Autodesk Inventor part; units mm, degrees
ref_plane "YZ Plane" through (0, 0, 0) normal (1, 0, 0) x (0, 1, 0)
ref_plane "XZ Plane" through (0, 0, 0) normal (0, 1, 0) x (-1, 0, 0)
ref_plane "XY Plane" through (0, 0, 0) normal (0, 0, 1) x (1, 0, 0)
sketch "Sketch_1" plane through (0, 0, 0) normal (0, 0, 1) x (1, 0, 0)
  line L0 (6, 0) -> (0, 0)
  line L1 (-0.8, 0) -> (-0.8, 2.7673)
  line L2 (-0.8, 2.7673) -> (-0.5333, 3.5)
  line L3 (-0.5333, 3.5) -> (0, 3.5)
  line L4 (0, 3.5) -> (0, 1.9)
  arc A0 (0, 1.9) -> (0.4, 1.5) centre (0.4, 1.9) ccw
  line L5 (0.4, 1.5) -> (6, 1.5)
  line L6 (6, 1.5) -> (6, 0)
  line L7 (6, 0) -> (-0.8, 0)
  line L8 (0, 0) -> (-0.8, 0)
  dimension "d6" = 6
revolve "Revolution1" add sketch "Sketch_1" angle 360 about axis through (6, 0, 0) along (1, 0, 0)
thread "Thread1"
sketch "Sketch_5" plane through (-0.05, 0, 0) normal (1, 0, 0) x (0, 0, -1)
  arc A0 (-0.6801, -0.1159) -> (-0.4404, -0.531) centre (-0.5499, -0.3175) ccw
  arc A1 (-0.341, -0.5357) -> (-0.4404, -0.531) centre (-0.3947, -0.62) ccw
  arc A2 (-0.341, -0.5357) -> (-0.2934, -0.5632) centre (0, 0) ccw
  arc A3 (-0.2397, -0.6469) -> (-0.2934, -0.5632) centre (-0.3396, -0.6519) ccw
  arc A4 (-0.2397, -0.6469) -> (0.2397, -0.6469) centre (0, -0.635) ccw
  arc A5 (0.2934, -0.5632) -> (0.2397, -0.6469) centre (0.3396, -0.6519) ccw
  arc A6 (0.2934, -0.5632) -> (0.341, -0.5357) centre (0, 0) ccw
  arc A7 (0.4404, -0.531) -> (0.341, -0.5357) centre (0.3947, -0.62) ccw
  arc A8 (0.4404, -0.531) -> (0.6801, -0.1159) centre (0.5499, -0.3175) ccw
  arc A9 (0.6344, -0.0275) -> (0.6801, -0.1159) centre (0.7343, -0.0318) ccw
  arc A10 (0.6344, -0.0275) -> (0.6344, 0.0275) centre (0, 0) ccw
  arc A11 (0.6801, 0.1159) -> (0.6344, 0.0275) centre (0.7343, 0.0318) ccw
  arc A12 (0.6801, 0.1159) -> (0.4404, 0.531) centre (0.5499, 0.3175) ccw
  arc A13 (0.341, 0.5357) -> (0.4404, 0.531) centre (0.3947, 0.62) ccw
  arc A14 (0.341, 0.5357) -> (0.2934, 0.5632) centre (0, 0) ccw
  arc A15 (0.2397, 0.6469) -> (0.2934, 0.5632) centre (0.3396, 0.6519) ccw
  arc A16 (0.2397, 0.6469) -> (-0.2397, 0.6469) centre (0, 0.635) ccw
  arc A17 (-0.2934, 0.5632) -> (-0.2397, 0.6469) centre (-0.3396, 0.6519) ccw
  arc A18 (-0.2934, 0.5632) -> (-0.341, 0.5357) centre (0, 0) ccw
  arc A19 (-0.4404, 0.531) -> (-0.341, 0.5357) centre (-0.3947, 0.62) ccw
  arc A20 (-0.4404, 0.531) -> (-0.6801, 0.1159) centre (-0.5499, 0.3175) ccw
  arc A21 (-0.6344, 0.0275) -> (-0.6801, 0.1159) centre (-0.7343, 0.0318) ccw
  arc A22 (-0.6344, 0.0275) -> (-0.6344, -0.0275) centre (0, 0) ccw
  arc A23 (-0.6801, -0.1159) -> (-0.6344, -0.0275) centre (-0.7343, -0.0318) ccw
extrude "Extrusion1" cut sketch "Sketch_5" against normal blind 0.75
sketch "Sketch_2" plane through (0, 0, 0) normal (0, 0, 1) x (1, 0, 0)
  line L0 (0.4552, 0) -> (0, 0)
  line L1 (-0.05, 0) -> (-0.05, 0.875)
  line L2 (-0.05, 0.875) -> (0.4552, 0)
  line L3 (0.4552, 0) -> (-0.05, 0)
revolve "Revolution2" cut sketch "Sketch_2" angle 360 about axis through (0.4552, 0, 0) along (1, 0, 0)
sketch "スケッチ4" plane through (6, 0, 0) normal (1, 0, 0) x (0, 0, -1)
  circle A0 centre (0, 0) radius 1.5
extrude "押し出し2" cut sketch "スケッチ4" against normal blind 2
sketch "スケッチ5" plane through (-0.8, 0, 0) normal (-1, 0, 0) x (0, 0, 1)
  arc A0 (0.4404, -0.531) -> (0.341, -0.5357) centre (0.3947, -0.62) ccw
  arc A1 (0.2934, -0.5632) -> (0.341, -0.5357) centre (0, 0) ccw
  arc A2 (0.2934, -0.5632) -> (0.2397, -0.6469) centre (0.3396, -0.6519) ccw
  arc A3 (-0.2397, -0.6469) -> (0.2397, -0.6469) centre (0, -0.635) ccw
  arc A4 (-0.2397, -0.6469) -> (-0.2934, -0.5632) centre (-0.3396, -0.6519) ccw
  arc A5 (-0.341, -0.5357) -> (-0.2934, -0.5632) centre (0, 0) ccw
  arc A6 (-0.341, -0.5357) -> (-0.4404, -0.531) centre (-0.3947, -0.62) ccw
  arc A7 (-0.6801, -0.1159) -> (-0.4404, -0.531) centre (-0.5499, -0.3175) ccw
  arc A8 (-0.6801, -0.1159) -> (-0.6344, -0.0275) centre (-0.7343, -0.0318) ccw
  arc A9 (-0.6344, 0.0275) -> (-0.6344, -0.0275) centre (0, 0) ccw
  arc A10 (-0.6344, 0.0275) -> (-0.6801, 0.1159) centre (-0.7343, 0.0318) ccw
  arc A11 (-0.4404, 0.531) -> (-0.6801, 0.1159) centre (-0.5499, 0.3175) ccw
  arc A12 (-0.4404, 0.531) -> (-0.341, 0.5357) centre (-0.3947, 0.62) ccw
  arc A13 (-0.2934, 0.5632) -> (-0.341, 0.5357) centre (0, 0) ccw
  arc A14 (-0.2934, 0.5632) -> (-0.2397, 0.6469) centre (-0.3396, 0.6519) ccw
  arc A15 (0.2397, 0.6469) -> (-0.2397, 0.6469) centre (0, 0.635) ccw
  arc A16 (0.2397, 0.6469) -> (0.2934, 0.5632) centre (0.3396, 0.6519) ccw
  arc A17 (0.341, 0.5357) -> (0.2934, 0.5632) centre (0, 0) ccw
  arc A18 (0.341, 0.5357) -> (0.4404, 0.531) centre (0.3947, 0.62) ccw
  arc A19 (0.6801, 0.1159) -> (0.4404, 0.531) centre (0.5499, 0.3175) ccw
  arc A20 (0.6801, 0.1159) -> (0.6344, 0.0275) centre (0.7343, 0.0318) ccw
  arc A21 (0.6344, -0.0275) -> (0.6344, 0.0275) centre (0, 0) ccw
  arc A22 (0.6344, -0.0275) -> (0.6801, -0.1159) centre (0.7343, -0.0318) ccw
  arc A23 (0.4404, -0.531) -> (0.6801, -0.1159) centre (0.5499, -0.3175) ccw
  circle A24 centre (0, 0) radius 2.7673
  arc A25 (-0.6801, -0.1159) -> (-0.7578, -0.4375) centre (-0.5499, -0.3175) ccw
  line L0 (-0.7578, -0.4375) -> (-0.7578, 0.4375)
  line L1 (-0.7578, 0.4375) -> (0, 0.875)
  line L2 (0, 0.875) -> (0.7578, 0.4375)
  line L3 (0.7578, 0.4375) -> (0.7578, -0.4375)
  line L4 (0.7578, -0.4375) -> (0, -0.875)
  line L5 (0, -0.875) -> (-0.7578, -0.4375)
  point P0 (-0.5499, -0.5575)
  point P1 (-0.2078, -0.755)
  point P2 (-0.7578, 0.1975)
  point P3 (-0.7578, -0.1975)
  point P4 (-0.2078, 0.755)
  point P5 (-0.5499, 0.5575)
  point P6 (0.5499, 0.5575)
  point P7 (0.2078, 0.755)
  point P8 (0.7578, -0.1975)
  point P9 (0.7578, 0.1975)
  point P10 (0.2078, -0.755)
  point P11 (0.5499, -0.5575)
  point P12 (-0.7578, 0.4375)
  point P13 (-0.7578, 0.4375)
  point P14 (0, 0.875)
  point P15 (0, 0.875)
  point P16 (0, -0.875)
  point P17 (0, -0.875)
extrude "押し出し3" cut sketch "スケッチ5" against normal up to surface (0.75 mm away) contours A23 L4 A3 A2 A1 A0 | A23 A22 A21 A20 A19 L3 | L5 A7 A6 A5 A4 A3 | A19 A18 A17 A16 A15 L2 | L0 A11 A10 A9 A8 A7 | A15 A14 A13 A12 A11 L1
extrude "押し出し4" add sketch "スケッチ5" against normal up to surface (0.75 mm away) contours L4 A23 | L3 A23 | A3 L4 | A3 L5 | L3 A19 | L2 A19 | A7 L5 | A7 L0 | L2 A15 | L1 A15 | A11 L0 | A11 L1
properties part number "超極低頭ネジL4M3" material "ステンレス鋼"
Verification items for the finished model (mm, model axes). A direction names the side the tool comes from. Round coordinates to 2 decimals unless told otherwise and drop trailing zeros. Write each loop counter-clockwise with the first axis right and the second up, starting at its lowest first coordinate (ties: lowest second). Pieces come first, ordered by that corner, then holes. Notation, with made-up numbers: (-6, 17) -> (14, 17) arc R19 cw to (14, 29) -> close; hole circle Ø7 at (78.25, 19). An arc over 180 degrees is marked (long way). Write each question's results on one line, items separated by ' | '. Start each with the question number.
1. Cross-section at A-A (x = 1.1). Enter the section's corners in (y, z), then the cut area to 3 significant figures.
2. Material ranges on probe 1 along Y at (x, z) = (-0.4, 0.25); probe 2 along X at (y, z) = (-1, 2); probe 3 along Z at (x, y) = (3, 0), recorded low to high. Write a range as from..to.
3. Depth check by flat-ended pin: P1, Ø1, axis at x = 2, z = -1, coming from the -Y side; P2, Ø4, axis at y = -2.5, z = 1.5, coming from the -X side. Enter the tip coordinate at first touch or a pass-through.
4. Set-up check for faces 1 (the flat face through (0, 2, -2)), 2 (the cylindrical face through (-0.263, 3.233, -1.341)): record each of +Z, -Z, +X, -X, +Y, -Y from which the full face is reachable in a straight line by a thin tool's end or side.
5. Cross-section at B-B (x = 0.2). Enter the section's corners in (y, z).
6. Draft check along Z on faces 3 (the flat face through (4, 0, 0)), 4 (the conical face through (0.367, -0.033, 0.148)), 5 (the cylindrical face through (2.23, -1.5, 0.07)). Enter one of: +Z half, -Z half, draft (parallel to the pull), parting line (faces both ways), or undercut.
Solutions:
1) outline: circle Ø3 at (0, 0) | area: 7.07 mm2
2) probe 1: y = -3.49..-0.73, 0.73..3.49 | probe 2: x = -0.8..0 | probe 3: z = -1.5..1.5
3) P1: stops at y = -1.41 | P2: stops at x = -0.8
4) face 1: +X | face 2: +X, -X
5) outline: circle Ø3.11 at (0, 0); hole circle Ø0.88 at (0, 0)
6) face 3: draft | face 4: undercut | face 5: parting line
